Check sheet for the modelled part. Datum: model origin and axes. Units: mm. Face numbers are marked on the shaded views. A direction names the side the tool comes from. Coordinates: 2 decimals unless noted, no trailing zeros. Loops run counter-clockwise (first coordinate to the right, second up) from the corner with the lowest first, then second, coordinate; pieces in that order, holes last. Notation, with made-up numbers: (-26.5, 64.5) -> (24.5, 64.5) arc R30 ccw to (24.5, 99.5) -> close; hole circle Ø9 at (80, 32). An arc over 180 degrees is marked (long way). Use CSV: the item, a comma, the result in double quotes.
Autodesk Inventor part; units mm, degrees
ref_plane "YZ Plane" through (0, 0, 0) normal (1, 0, 0) x (0, 1, 0)
ref_plane "XZ Plane" through (0, 0, 0) normal (0, 1, 0) x (-1, 0, 0)
ref_plane "XY Plane" through (0, 0, 0) normal (0, 0, 1) x (1, 0, 0)
sketch "Sketch1" plane through (0, 0, 0) normal (0, 1, 0) x (-1, 0, 0)
  line L0 (0, 0) -> (326.2264, 0) construction
  line L1 (326.2264, 0) -> (326.2264, -146.0251) construction
  line L2 (326.2264, -146.0251) -> (0, -146.0251) construction
  line L3 (0, -146.0251) -> (0, 0) construction
  line L4 (67.2736, -57.5928) -> (73.4159, -57.5928)
  line L5 (73.4159, -57.5928) -> (73.4159, -51.4505)
  line L6 (73.4159, -51.4505) -> (85.7005, -51.4505)
  line L7 (85.7005, -51.4505) -> (85.7005, -57.5928)
  line L8 (85.7005, -57.5928) -> (91.8428, -57.5928)
  line L9 (91.8428, -57.5928) -> (91.8428, -63.7351)
  line L10 (91.8428, -63.7351) -> (97.9851, -63.7351)
  line L11 (97.9851, -63.7351) -> (97.9851, -57.5928)
  line L12 (97.9851, -57.5928) -> (104.1274, -57.5928)
  line L13 (104.1274, -57.5928) -> (104.1274, -51.4505)
  line L14 (104.1274, -51.4505) -> (116.412, -51.4505)
  line L15 (116.412, -51.4505) -> (116.412, -45.3082)
  line L16 (116.412, -45.3082) -> (110.2697, -45.3082)
  line L17 (110.2697, -45.3082) -> (110.2697, -39.1659)
  line L18 (110.2697, -39.1659) -> (104.1274, -39.1659)
  line L19 (104.1274, -39.1659) -> (104.1274, -33.0236)
  line L20 (104.1274, -33.0236) -> (97.9851, -33.0236)
  line L21 (97.9851, -33.0236) -> (97.9851, -26.8813)
  line L22 (97.9851, -26.8813) -> (85.7005, -26.8813)
  line L23 (85.7005, -26.8813) -> (85.7005, -20.739)
  line L24 (69.1807, -19.7772) -> (85.7005, -19.7772)
  line L25 (85.7005, -19.7772) -> (85.7005, -20.739)
  line L26 (67.2736, -57.5928) -> (61.1313, -57.5928)
  line L27 (61.1313, -57.5928) -> (61.1313, -51.4505)
  line L28 (61.1313, -51.4505) -> (48.8467, -51.4505)
  line L29 (48.8467, -51.4505) -> (48.8467, -57.5928)
  line L30 (48.8467, -57.5928) -> (42.7043, -57.5928)
  line L31 (42.7043, -57.5928) -> (42.7043, -63.7351)
  line L32 (42.7043, -63.7351) -> (36.562, -63.7351)
  line L33 (36.562, -63.7351) -> (36.562, -57.5928)
  line L34 (36.562, -57.5928) -> (30.4197, -57.5928)
  line L35 (30.4197, -57.5928) -> (30.4197, -51.4505)
  line L36 (30.4197, -51.4505) -> (20.0422, -51.4505)
  line L37 (20.0422, -51.4505) -> (20.0422, -45.3082)
  line L38 (20.0422, -45.3082) -> (26.1845, -45.3082)
  line L39 (26.1845, -45.3082) -> (26.1845, -39.1659)
  line L40 (26.1845, -39.1659) -> (32.3268, -39.1659)
  line L41 (32.3268, -39.1659) -> (32.3268, -33.0236)
  line L42 (32.3268, -33.0236) -> (38.4691, -33.0236)
  line L43 (38.4691, -33.0236) -> (38.4691, -26.8813)
  line L44 (38.4691, -26.8813) -> (50.7538, -26.8813)
  line L45 (50.7538, -26.8813) -> (50.7538, -20.739)
  line L46 (69.1807, -19.7772) -> (50.7538, -19.7772)
  line L47 (50.7538, -19.7772) -> (50.7538, -20.739)
  line L48 (39.2885, -39.7662) -> (39.2885, -44.5453)
  line L49 (39.2885, -44.5453) -> (44.0675, -44.5453)
  line L50 (44.0675, -44.5453) -> (44.0675, -39.7662)
  line L51 (44.0675, -39.7662) -> (39.2885, -39.7662)
  line L52 (56.9879, -39.7662) -> (56.9879, -44.5453)
  line L53 (56.9879, -44.5453) -> (61.7669, -44.5453)
  line L54 (56.9879, -39.7662) -> (61.7669, -39.7662)
  line L55 (61.7669, -39.7662) -> (61.7669, -44.5453)
  line L56 (74.6873, -39.7662) -> (79.4663, -39.7662)
  line L57 (79.4663, -39.7662) -> (79.4663, -44.5453)
  line L58 (79.4663, -44.5453) -> (74.6873, -44.5453)
  line L59 (74.6873, -44.5453) -> (74.6873, -39.7662)
  line L60 (92.3867, -39.7662) -> (97.1657, -39.7662)
  line L61 (97.1657, -39.7662) -> (97.1657, -44.5453)
  line L62 (97.1657, -44.5453) -> (92.3867, -44.5453)
  line L63 (92.3867, -44.5453) -> (92.3867, -39.7662)
  dimension "d3" = 6.1423
  dimension "d6" = 6.1423
  dimension "d7" = 6.1423
  dimension "d8" = 6.1423
  dimension "d9" = 6.1423
  dimension "d10" = 6.1423
  dimension "d11" = 6.1423
  dimension "d12" = 6.1423
  dimension "d13" = 12.2846
  dimension "d14" = 12.2846
  dimension "d15" = 6.1423
  dimension "d16" = 6.1423
  dimension "d17" = 6.1423
  dimension "d18" = 6.1423
  dimension "d19" = 6.1423
  dimension "d20" = 12.2846
  dimension "d21" = 6.1423
  dimension "d22" = 6.1423
  dimension "d23" = 6.1423
  dimension "d29" = 12.9204
  dimension "d30" = 12.9204
  dimension "d31" = 13.104
  dimension "d32" = 13.104
  dimension "d33" = 12.9204
  dimension "d34" = 4.779
  dimension "d35" = 4.779
  dimension "d36" = 4.779
  dimension "d37" = 4.779
  dimension "d38" = 4.779
  dimension "d39" = 4.779
  dimension "d40" = 4.779
extrude "Extrusion1" add sketch "Sketch1" along normal blind 6.35
equation "\"d6\" = d3"
equation "\"d7\" = d6"
equation "\"d8\" = d3"
equation "\"d9\" = d7"
equation "\"d10\" = d7"
equation "\"d11\" = d10"
equation "\"d12\" = d6"
equation "\"d13\" = 2 * d3"
equation "\"d14\" = d13"
equation "\"d15\" = d6"
equation "\"d16\" = d11"
equation "\"d17\" = d16"
equation "\"d18\" = d17"
equation "\"d19\" = d17"
equation "\"d20\" = d13"
equation "\"d23\" = 0.5 * d13"
equation "\"d30\" = d29"
equation "\"d32\" = d31"
equation "\"d33\" = d30"
equation "\"d35\" = d34"
equation "\"d37\" = d35"
equation "\"d38\" = d36"
equation "\"d40\" = d38"
properties part number "Monster1"
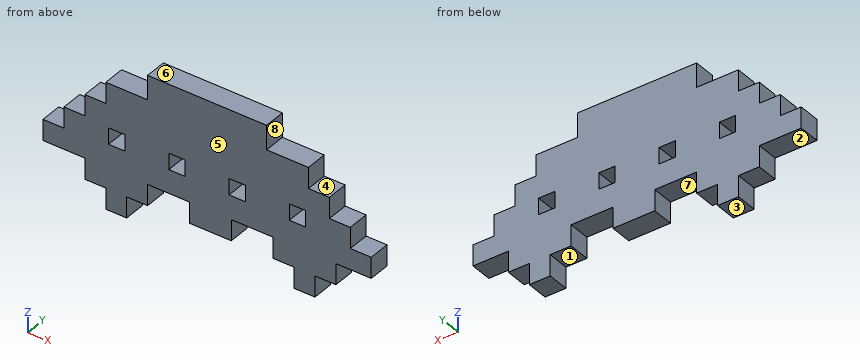
1) Cross-section at B-B on x = -76.5. Record the boundary of the cut face in (y, z), and give its area (3 significant figures).
Answer below:
outline,"(0, -51.45) -> (6.35, -51.45) -> (6.35, -44.55) -> (0, -44.55) -> close; (0, -39.77) -> (6.35, -39.77) -> (6.35, -19.78) -> (0, -19.78) -> close"
area,"171 mm²"
2) Thickness scan on line 1 along X through (y, z) = (1, -44.5); line 2 along X through (y, z) = (6.25, -57); line 3 along Z through (x, y) = (-44, 4.5). Record the ranges inside material, lowest first. Write a range as from..to.
Answer below:
line 1,"x = -110.27..-97.17, -92.39..-79.47, -74.69..-61.77, -56.99..-44.07, -39.29..-26.18"
line 2,"x = -104.13..-85.7, -73.42..-61.13, -48.85..-30.42"
line 3,"z = -57.59..-44.55, -39.77..-26.88"
3) Go/stop test with flat-tipped pins: pin 1 Ø1 at (x, y) = (-88, 1) entering from +Z; pin 2 Ø1.8 at (y, z) = (2.5, -53.5) entering from +X; pin 3 Ø2.5 at (x, y) = (-77.5, 2) entering from -Z. Record where each tip stops, or that it passes through.
Answer below:
pin 1,"stops at z = -26.88"
pin 2,"stops at x = -30.42"
pin 3,"stops at z = -51.45"
4) Cross-section at D-D on x = -54. Record the boundary of the cut face in (y, z), and give its area (3 significant figures).
Answer below:
outline,"(0, -51.45) -> (6.35, -51.45) -> (6.35, -19.78) -> (0, -19.78) -> close"
area,"201 mm²"
5) Access from +Z, -Z, +X, -X, +Y, -Y to the whole of each face (thin tool, end or side, straight path). Record for the marked faces 1, 2, 3, 4 and 5.
Answer below:
face 1,"-Z, +Y, -Y"
face 2,"-Z, -X, +Y, -Y"
face 3,"-Z, +X, -X, +Y, -Y"
face 4,"+Z, +X, +Y, -Y"
face 5,"+Z, -Z, +X, -X, -Y"
6) Cross-section at C-C on y = 5. Give the number of separate pieces and of enclosed holes in the cut face, and give its area (3 significant figures).
Answer below:
separate pieces,"1"
enclosed holes,"4"
area,"2,450 mm²"
7) Draft check along X on the marked faces 6, 7 and 8. Enter one of: released by +X, released by -X, zero draft, split by the parting line, or undercut.
Answer below:
face 6,"zero draft"
face 7,"undercut"
face 8,"released by +X"
8) Cross-section at A-A on z = -43. Record the boundary of the cut face in (x, y), and give its area (3 significant figures).
Answer below:
outline,"(-110.27, 0) -> (-97.17, 0) -> (-97.17, 6.35) -> (-110.27, 6.35) -> close; (-92.39, 0) -> (-79.47, 0) -> (-79.47, 6.35) -> (-92.39, 6.35) -> close; (-74.69, 0) -> (-61.77, 0) -> (-61.77, 6.35) -> (-74.69, 6.35) -> close; (-56.99, 0) -> (-44.07, 0) -> (-44.07, 6.35) -> (-56.99, 6.35) -> close; (-39.29, 0) -> (-26.18, 0) -> (-26.18, 6.35) -> (-39.29, 6.35) -> close"
area,"413 mm²"
